For this review, take the finished solid that the model builds, in its own axes (mm). A direction names the side the tool comes from. Coordinates: 2 decimals unless noted, no trailing zeros. Write each loop counter-clockwise with the first axis right and the second up, starting at its lowest first coordinate (ties: lowest second). Pieces come first, ordered by that corner, then holes. Notation, with made-up numbers: M 4.25,-7 L 51.25,-7 A27 ccw 51.25,12 Z; hole C 0.5,-3.5 d1. An arc over 180 degrees is marked long. One line per question, with ' | ' between items.
from build123d import *

# Parameters (mm, degrees)
BOSS_EXTRU_1_DEPTH      = 20
CONG_1_R                = 2.38125
ESQUISSE2_W             = 63.5
ESQUISSE2_H             = 35.56
BOSS_EXTRU_2_DEPTH      = 5.08
EMPREINTE1_START        = -25.08
EMPREINTE1_DEPTH        = 5.08
D_PLACER_START          = -25.08
D_PLACER_LA_FACE1_DEPTH = 5.08
EMPREINTE4_START        = 17.46
EMPREINTE4_DEPTH        = 2.54
D_PLACER_START_2        = 16.952
D_PLACER_LA_FACE2_DEPTH = 3.048
CHANFREIN1_SIZE         = 6.35
CHANFREIN1_SIZE2        = 3.81
CHANFREIN2_SIZE         = 3.81
CHANFREIN2_SIZE2        = 6.35
BOSS_EXTRU_3_DEPTH      = 45.08
ESQUISSE4_W             = 44.45
ESQUISSE4_H             = 22.86
ENL_V_MAT_EXTRU_1_DEPTH = 38.1
ESQUISSE5_W             = 12.7
ESQUISSE5_H             = 3.81
BOSS_EXTRU_4_DEPTH      = 12.7
CONG_2_R                = 2.54
D_GAGEMENT_61_D         = 3.7973
ENL_V_START             = -38.1
ENL_V_MAT_EXTRU_2_DEPTH = 119.894566185
D_GAGEMENT_62_D         = 3.7973
D_GAGEMENT_62_DEPTH     = 18.796
D_GAGEMENT_62_TIP       = 1.140824014


# Read off the part's stored shape, not the designer's step: Empreinte1, Déplacer la face1, Empreinte4, Déplacer la face2
with BuildPart() as part:
    # Esquisse1 → Boss.-Extru.1 (new, symmetric)
    with BuildSketch(Plane.XY):
        Polygon((-31.75, -1.905), (-31.75, 33.655), (31.75, 33.655), (31.75, -1.905), (12.92225, -1.905), (12.92225, 4.445), (13.87475, 5.3975), (21.59, 5.3975), (21.59, 21.59), (-21.59, 21.59), (-21.59, 5.3975), (-13.87475, 5.3975), (-12.92225, 4.445), (-12.92225, -1.905), align=None)
    extrude(amount=BOSS_EXTRU_1_DEPTH, both=True)

    # Congé1
    cong_1_edges = [part.edges().sort_by_distance(p)[0] for p in [
        (21.59, 5.3975, 0),
        (21.59, 21.59, 0),
        (-21.59, 21.59, 0),
        (-21.59, 5.3975, 0),
    ]]
    fillet(cong_1_edges, radius=CONG_1_R)

    # Esquisse2 → Boss.-Extru.2 (add)
    with BuildSketch(Plane(origin=(0, 0, -20), x_dir=(-1, 0, 0), z_dir=(0, 0, -1))):
        with Locations((0, 15.875)):
            Rectangle(ESQUISSE2_W, ESQUISSE2_H)
    extrude(amount=BOSS_EXTRU_2_DEPTH)

    # Empreinte1 outline → Empreinte1 (cut)
    with BuildSketch(Plane.XY.offset(EMPREINTE1_START)):
        with BuildLine():
            Line((14.44625, 7.9375), (16.66875, 7.9375))
            ThreePointArc((16.66875, 7.9375), (17.366201977, 9.621298023), (19.05, 10.31875))
            Line((19.05, 10.31875), (19.05, 16.66875))
            ThreePointArc((19.05, 16.66875), (17.366201977, 17.366201977), (16.66875, 19.05))
            Line((16.66875, 19.05), (-16.66875, 19.05))
            ThreePointArc((-16.66875, 19.05), (-17.366201977, 17.366201977), (-19.05, 16.66875))
            Line((-19.05, 16.66875), (-19.05, 10.31875))
            ThreePointArc((-19.05, 10.31875), (-17.366201977, 9.621298023), (-16.66875, 7.9375))
            Line((-16.66875, 7.9375), (-14.44625, 7.9375))
            Line((-14.44625, 7.9375), (-11.90625, 5.3975))
            Line((-11.90625, 5.3975), (-11.90625, -1.905))
            Line((-11.90625, -1.905), (11.90625, -1.905))
            Line((11.90625, -1.905), (11.90625, 5.3975))
            Line((11.90625, 5.3975), (14.44625, 7.9375))
        make_face()
    extrude(amount=EMPREINTE1_DEPTH, mode=Mode.SUBTRACT)

    # Déplacer la face1 outline → Déplacer la face1 (cut)
    with BuildSketch(Plane.XY.offset(D_PLACER_START)):
        with BuildLine():
            Line((-14.867090979, 6.9215), (-12.92225, 4.976659021))
            Line((-12.92225, 4.976659021), (-12.92225, -1.905))
            Line((-12.92225, -1.905), (-11.90625, -1.905))
            Line((-11.90625, -1.905), (-11.90625, 5.3975))
            Line((-11.90625, 5.3975), (-14.44625, 7.9375))
            Line((-14.44625, 7.9375), (-16.66875, 7.9375))
            ThreePointArc((-16.66875, 7.9375), (-17.366201977, 9.621298023), (-19.05, 10.31875))
            Line((-19.05, 10.31875), (-19.05, 16.66875))
            ThreePointArc((-19.05, 16.66875), (-17.366201977, 17.366201977), (-16.66875, 19.05))
            Line((-16.66875, 19.05), (16.66875, 19.05))
            ThreePointArc((16.66875, 19.05), (17.366201977, 17.366201977), (19.05, 16.66875))
            Line((19.05, 16.66875), (19.05, 10.31875))
            ThreePointArc((19.05, 10.31875), (17.366201977, 9.621298023), (16.66875, 7.9375))
            Line((16.66875, 7.9375), (14.44625, 7.9375))
            Line((14.44625, 7.9375), (11.90625, 5.3975))
            Line((11.90625, 5.3975), (11.90625, -1.905))
            Line((11.90625, -1.905), (12.92225, -1.905))
            Line((12.92225, -1.905), (12.92225, 4.976659021))
            Line((12.92225, 4.976659021), (14.867090979, 6.9215))
            Line((14.867090979, 6.9215), (18.13805068, 6.9215))
            ThreePointArc((18.13805068, 6.9215), (18.084622467, 8.902877533), (20.066, 8.84944932))
            Line((20.066, 8.84944932), (20.066, 18.13805068))
            ThreePointArc((20.066, 18.13805068), (18.084622467, 18.084622467), (18.13805068, 20.066))
            Line((18.13805068, 20.066), (-18.13805068, 20.066))
            ThreePointArc((-18.13805068, 20.066), (-18.084622467, 18.084622467), (-20.066, 18.13805068))
            Line((-20.066, 18.13805068), (-20.066, 8.84944932))
            ThreePointArc((-20.066, 8.84944932), (-18.084622467, 8.902877533), (-18.13805068, 6.9215))
            Line((-18.13805068, 6.9215), (-14.867090979, 6.9215))
        make_face()
    extrude(amount=D_PLACER_LA_FACE1_DEPTH, mode=Mode.SUBTRACT)

    # Empreinte4 outline → Empreinte4 (cut)
    with BuildSketch(Plane.XY.offset(EMPREINTE4_START)):
        with BuildLine():
            ThreePointArc((-27.94, 7.62), (-26.67, 6.35), (-25.4, 7.62))
            Line((-25.4, 7.62), (-25.4, 20.32))
            ThreePointArc((-25.4, 20.32), (-26.67, 21.59), (-27.94, 20.32))
            Line((-27.94, 20.32), (-27.94, 7.62))
        make_face()
        with BuildLine():
            Line((25.4, 20.32), (25.4, 7.62))
            ThreePointArc((25.4, 7.62), (26.67, 6.35), (27.94, 7.62))
            Line((27.94, 7.62), (27.94, 20.32))
            ThreePointArc((27.94, 20.32), (26.67, 21.59), (25.4, 20.32))
        make_face()
    extrude(amount=EMPREINTE4_DEPTH, mode=Mode.SUBTRACT)

    # Déplacer la face2 outline → Déplacer la face2 (cut)
    with BuildSketch(Plane.XY.offset(D_PLACER_START_2)):
        with BuildLine():
            ThreePointArc((-28.448, 7.62), (-26.67, 5.842), (-24.892, 7.62))
            Line((-24.892, 7.62), (-24.892, 20.32))
            ThreePointArc((-24.892, 20.32), (-26.67, 22.098), (-28.448, 20.32))
            Line((-28.448, 20.32), (-28.448, 7.62))
        make_face()
        with BuildLine():
            Line((24.892, 20.32), (24.892, 7.62))
            ThreePointArc((24.892, 7.62), (26.67, 5.842), (28.448, 7.62))
            Line((28.448, 7.62), (28.448, 20.32))
            ThreePointArc((28.448, 20.32), (26.67, 22.098), (24.892, 20.32))
        make_face()
    extrude(amount=D_PLACER_LA_FACE2_DEPTH, mode=Mode.SUBTRACT)

    # Chanfrein1
    chanfrein1_edges = [part.edges().sort_by_distance(p)[0] for p in [
        (-12.92225, -1.905, -2.54),
    ]]
    chanfrein1_side = [part.faces().sort_by_distance(p)[0] for p in [
        (-22.336125, -1.905, -2.54),
    ]]
    chamfer(chanfrein1_edges, length=CHANFREIN1_SIZE, length2=CHANFREIN1_SIZE2, reference=chanfrein1_side[0])

    # Chanfrein2
    chanfrein2_edges = [part.edges().sort_by_distance(p)[0] for p in [
        (12.92225, -1.905, -2.54),
    ]]
    chanfrein2_side = [part.faces().sort_by_distance(p)[0] for p in [
        (12.92225, 1.302160596, -2.726935132),
    ]]
    chamfer(chanfrein2_edges, length=CHANFREIN2_SIZE, length2=CHANFREIN2_SIZE2, reference=chanfrein2_side[0])

    # Esquisse3 → Boss.-Extru.3 (add)
    with BuildSketch(Plane.XY.offset(20)):
        Polygon((-31.75, -1.905), (-31.75, -59.055), (31.75, -59.055), (31.75, -1.905), (22.225, -1.905), (22.225, -24.765), (-22.225, -24.765), (-22.225, -1.905), align=None)
    extrude(amount=-BOSS_EXTRU_3_DEPTH)

    # Esquisse4 → Enlèv. mat.-Extru.1 (cut)
    with BuildSketch(Plane.XY.offset(20)):
        with Locations((0, -36.195)):
            Rectangle(ESQUISSE4_W, ESQUISSE4_H)
    extrude(amount=-ENL_V_MAT_EXTRU_1_DEPTH, mode=Mode.SUBTRACT)

    # Esquisse5 → Boss.-Extru.4 (add)
    with BuildSketch(Plane(origin=(0, 0, -25.08), x_dir=(-1, 0, 0), z_dir=(0, 0, -1))):
        with Locations((0, -27.519)):
            Rectangle(ESQUISSE5_W, ESQUISSE5_H)
    extrude(amount=BOSS_EXTRU_4_DEPTH)

    # Congé2
    cong_2_edges = [part.edges().sort_by_distance(p)[0] for p in [
        (6.35, -27.519, -37.78),
        (-6.35, -27.519, -37.78),
    ]]
    fillet(cong_2_edges, radius=CONG_2_R)

    # Dégagement #61 (through all)
    with Locations(Plane(origin=(0, -25.614, 0), x_dir=(1, 0, 0), z_dir=(0, 1, 0))):
        with Locations((0, 31.43)):
            Hole(D_GAGEMENT_61_D / 2)

    # Esquisse8 → Enlèv. mat.-Extru.2 (cut)
    with BuildSketch(Plane(origin=(0, 0, -25.08), x_dir=(-1, 0, 0), z_dir=(0, 0, -1)).offset(ENL_V_START)):
        Polygon((266.493356743, 33.655), (31.75, 33.655), (22.86, 33.655), (22.86, 28.575), (26.67, 24.765), (31.75, 24.765), (266.493356743, 24.765), (735.980070228, 24.765), (735.980070228, 33.655), align=None)
    enl_v_mat_extru_2 = extrude(amount=ENL_V_MAT_EXTRU_2_DEPTH, mode=Mode.SUBTRACT)

    # Symétrie1: Enlèv. mat.-Extru.2 across plane
    add(enl_v_mat_extru_2.mirror(Plane(origin=(0, 0, 0), x_dir=(0, 0, 1), z_dir=(1, 0, 0))), mode=Mode.SUBTRACT)

    # Dégagement #62
    with Locations(Plane(origin=(0, 0, 13.02), x_dir=(-1, 0, 0), z_dir=(0, 0, -1))):
        with Locations((27.94, 29.845), (-27.94, 29.845)):
            Hole(D_GAGEMENT_62_D / 2, depth=D_GAGEMENT_62_DEPTH)
            with Locations((0, 0, -(D_GAGEMENT_62_DEPTH + D_GAGEMENT_62_TIP / 2))):  # 118° drill point
                Cone(0, D_GAGEMENT_62_D / 2, D_GAGEMENT_62_TIP, mode=Mode.SUBTRACT)


solid = part.part
1. Clearance check with flat-ended pins moving along their axes: P1, Ø4.5, axis at x = 27, y = 31, coming from the -Z side; P2, Ø3, axis at y = -28, z = -28, coming from the -X side; P3, Ø4, axis at x = 30, z = -7.5, coming from the +Y side (3 decimals); P4, Ø6, axis at x = 11.5, y = -3.5, coming from the +Z side. State where each tip first meets the part, or that it passes through.
Computed values:
P1: stops at z = 13.02 | P2: stops at x = -6.35 | P3: stops at y = 24.765 | P4: passes through
2. Take a section at A-A on x = -10. State the section outline as (y, z) points (3 decimals).
Computed values:
outline: M -59.055,-25.08 L -24.765,-25.08 L -24.765,-18.1 L -47.625,-18.1 L -47.625,20 L -59.055,20 Z; M 20.066,-25.08 L 33.655,-25.08 L 33.655,20 L 21.59,20 L 21.59,-20 L 20.066,-20 Z
3. Take a section at B-B on y = -4. State the section outline as (x, z) points (3 decimals).
Computed values:
outline: M -31.75,-25.08 L -22.225,-25.08 L -22.225,20 L -31.75,20 Z; M 22.225,-25.08 L 31.75,-25.08 L 31.75,20 L 22.225,20 Z
4. Draft analysis for pull direction X (two halves, no side actions). For faces 6 (the flat face through (0, -59.055, -2)), 7 (the cylindrical face through (20.874, 20.911, -0.28)), state which applies: pulls with the +X half, pulls with the -X half, needs draft (parallel to the pull), parting line crosses it, or undercut.
Computed values:
face 6: needs draft | face 7: undercut
5. Take a section at C-C on x = 0. State the section outline as (y, z) points (3 decimals), plus the area to 3 significant figures.
Computed values:
outline: M -59.055,-25.08 L -29.424,-25.08 L -29.424,-29.531 L -25.614,-29.531 L -25.614,-25.08 L -24.765,-25.08 L -24.765,-18.1 L -47.625,-18.1 L -47.625,20 L -59.055,20 Z; M -29.424,-37.78 L -25.614,-37.78 L -25.614,-33.329 L -29.424,-33.329 Z; M 20.066,-25.08 L 33.655,-25.08 L 33.655,20 L 21.59,20 L 21.59,-20 L 20.066,-20 Z | area: 1,260 mm2
6. Machinability: for faces 1 (the flat face through (-26, 28, 13.02)), 2 (the flat face through (0, 21.59, 0)), 3 (the flat face through (0, 33.655, -2)), 4 (the flat face through (21, -1.905, -2)), 5 (the flat face through (2, -29.424, -30)), which of the approach directions +Z, -Z, +X, -X, +Y, -Y give a long, thin tool a straight path to every point of the face, cutting with its end or side? Answer none if there is none.
Computed values:
face 1: -Z, -X, +Y | face 2: +Z | face 3: +Z, -Z, +X, -X, +Y | face 4: +Z, -Z | face 5: -Z, +X, -X, -Y
7. For line 1 along Y through (x, z) = (3, -12) (3 decimals); line 2 along Y through (x, z) = (3, -22) (3 decimals); line 3 along Y through (x, z) = (-18.5, -23.5) (3 decimals), list the stretches that pass through material, from the lowest coordinate up.
Computed values:
line 1: y = -59.055 to -47.625, 21.59 to 33.655 | line 2: y = -59.055 to -24.765, 20.066 to 33.655 | line 3: y = -59.055 to -24.765, -1.442 to 9.187, 17.8 to 33.655
